Part model, mm, in its own coordinate system. Face numbers are marked on the shaded views. A direction names the side the tool comes from. Give positions to 0.01 mm unless a question says otherwise; leave off trailing zeros. Order: outer loops, then holes, each group sorted by start corner. A loop starts at its lowest first (then second) coordinate and runs counter-clockwise, first axis right, second up. Notation, with made-up numbers: (48, 85) - (64, 85) arc R8 cw to (64, 93) - close; hole circle Ø5 at (57, -35.5). An arc over 180 degrees is marked (long way). One line per item, written item: value.
```python
from build123d import *

# Parameters (mm, degrees)
BOSS_EXTRUDE1_DEPTH  = 12
M3_CLEARANCE_HOLE1_D = 3.6


with BuildPart() as part:
    # Sketch2 → Boss-Extrude1 (new body)
    with BuildSketch(Plane(origin=(-74.202720672, 5.306098308, 687.991999443), x_dir=(0.9999999999999999, 0, -2.239969215025861e-08), z_dir=(2.239969215025861e-08, 0, 0.9999999999999999))):
        with BuildLine():
            Line((59.700000081, 87.500000033), (59.700000081, 88.000000033))
            Line((59.700000081, 88.000000033), (59.700000142, 107.000000033))
            ThreePointArc((59.700000142, 107.000000033), (59.905025396, 107.494974779), (60.400000144, 107.70000003))
            Line((60.400000144, 107.70000003), (99.800000144, 107.699999904))
            ThreePointArc((99.800000144, 107.699999904), (100.29497489, 107.49497465), (100.500000142, 106.999999902))
            Line((100.500000142, 106.999999902), (100.500000081, 87.999999902))
            Line((100.500000081, 87.999999902), (100.500000081, 87.499999902))
            Line((100.500000081, 87.499999902), (113.600000142, 87.49999986))
            Line((113.600000142, 87.49999986), (113.600000142, 89.49999986))
            Line((113.600000142, 89.49999986), (102.500000086, 89.49999986))
            Line((102.500000086, 89.49999986), (102.500000142, 106.999999896))
            ThreePointArc((102.500000142, 106.999999896), (101.709188457, 108.909188207), (99.80000015, 109.699999904))
            Line((99.80000015, 109.699999904), (60.40000015, 109.70000003))
            ThreePointArc((60.40000015, 109.70000003), (58.490811839, 108.909188346), (57.700000142, 107.000000039))
            Line((57.700000142, 107.000000039), (57.700000142, 89.500000075))
            Line((57.700000142, 89.500000075), (46.600000142, 89.500000075))
            Line((46.600000142, 89.500000075), (46.600000142, 87.500000075))
            Line((46.600000142, 87.500000075), (59.700000081, 87.500000033))
        make_face()
    extrude(amount=BOSS_EXTRUDE1_DEPTH)

    # M3 Clearance Hole1 (through all)
    with Locations(Plane(origin=(0, 94.806098383, 0), x_dir=(1, 0, 0), z_dir=(0, 1, 0))):
        with Locations((-24.202720482, -691.491998323), (35.797279518, -691.491996979)):
            Hole(M3_CLEARANCE_HOLE1_D / 2)


solid = part.part
```
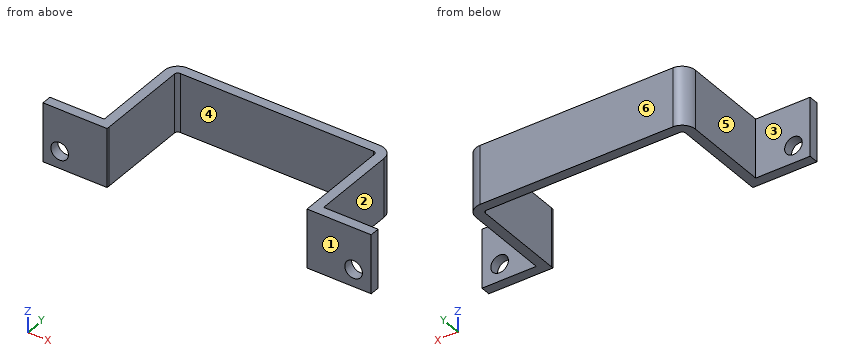
1) Drop flat-ended pins along their axis: P1, Ø6, axis at x = 18.5, y = 111.5, coming from the -Z side; P2, Ø3, axis at x = 13, z = 697, coming from the -Y side; P3, Ø3.5, axis at y = 101, z = 693, coming from the -X side; P4, Ø5, axis at y = 112, z = 690, coming from the +X side. Give the stop position or say it passes through.
Answer:
P1: stops at z = 687.99
P2: stops at y = 113.01
P3: stops at x = -16.5
P4: stops at x = 28.3
2) Slice it at B-B on z = 695.25. Write the cut outline in (x, y), then the cut area to 3 significant figures.
Answer:
outline: (-27.6, 92.81) - (-14.5, 92.81) - (-14.5, 112.31) arc R0.7 cw to (-13.8, 113.01) - (25.6, 113.01) arc R0.7 cw to (26.3, 112.31) - (26.3, 92.81) - (39.4, 92.81) - (39.4, 94.81) - (28.3, 94.81) - (28.3, 112.31) arc R2.7 ccw to (25.6, 115.01) - (-13.8, 115.01) arc R2.7 ccw to (-16.5, 112.31) - (-16.5, 94.81) - (-27.6, 94.81) - close
area: 212 mm2
3) Slice it at C-C on x = 35.5. Write the cut outline in (y, z), then the cut area to 3 significant figures.
Answer:
outline: (92.81, 687.99) - (94.81, 687.99) - (94.81, 689.72) - (92.81, 689.72) - close; (92.81, 693.27) - (94.81, 693.27) - (94.81, 699.99) - (92.81, 699.99) - close
area: 16.9 mm2
4) Which spindle directions (+Z, -Z, +X, -X, +Y, -Y) get a long thin tool onto all of the face, cutting with end or side? Do the marked faces 1, 2 and 3. Say none if no direction does.
Answer:
face 1: +Z, -Z, +X, -X, -Y
face 2: +Z, -Z, +X, +Y
face 3: +Z, -Z, -X, +Y
5) Two-plate mould, pull along X, no slides. Class the marked faces 4, 5 and 6: pulls with the +X half, pulls with the -X half, needs draft (parallel to the pull), parting line crosses it, or undercut.
Answer:
face 4: undercut
face 5: pulls with the -X half
face 6: needs draft
6) Slice it at D-D on z = 692.25. Write the cut outline in (x, y).
Answer:
outline: (-27.6, 92.81) - (-25.84, 92.81) - (-25.84, 94.81) - (-27.6, 94.81) - close; (-22.57, 92.81) - (-14.5, 92.81) - (-14.5, 112.31) arc R0.7 cw to (-13.8, 113.01) - (25.6, 113.01) arc R0.7 cw to (26.3, 112.31) - (26.3, 92.81) - (34.16, 92.81) - (34.16, 94.81) - (28.3, 94.81) - (28.3, 112.31) arc R2.7 ccw to (25.6, 115.01) - (-13.8, 115.01) arc R2.7 ccw to (-16.5, 112.31) - (-16.5, 94.81) - (-22.57, 94.81) - close; (37.43, 92.81) - (39.4, 92.81) - (39.4, 94.81) - (37.43, 94.81) - close
7) Slice it at A-A on y = 110.75. Write the cut outline in (x, z).
Answer:
outline: (-16.5, 687.99) - (-14.5, 687.99) - (-14.5, 699.99) - (-16.5, 699.99) - close; (26.3, 687.99) - (28.3, 687.99) - (28.3, 699.99) - (26.3, 699.99) - close
8) Wall check: line 1 along X through (y, z) = (96.75, 688.5); line 2 along X through (y, z) = (94, 698); line 3 along Y through (x, z) = (12, 699.25). Give the ranges that are in metal, low to high. Write a range as [from, to].
Answer:
line 1: x = [-16.5, -14.5], [26.3, 28.3]
line 2: x = [-27.6, -14.5], [26.3, 39.4]
line 3: y = [113.01, 115.01]
